```python
from build123d import *

# Parameters (mm, degrees)
SKETCH1_R                = 10
BOSS_EXTRUDE1_DEPTH      = 10
BOSS_EXTRUDE1_DEPTH_BACK = 10
SKETCH11_R               = 12.675
BOSS_EXTRUDE2_DEPTH      = 40
BOSS_EXTRUDE2_DEPTH_BACK = 40
SKETCH12_R               = 10.5
CUT_EXTRUDE6_DEPTH       = 81.0000001
SKETCH2_R                = 4.825
CUT_EXTRUDE7_DEPTH       = 30
LPATTERN1_COUNT          = 4
LPATTERN1_PITCH          = 4
LPATTERN2_COUNT          = 4
LPATTERN2_PITCH          = 4


with BuildPart() as part:
    # Sketch1 → Boss-Extrude1 (new body, two sides)
    with BuildSketch(Plane(origin=(0, 0, 0), x_dir=(0, 0, -1), z_dir=(1, 0, 0))) as boss_extrude1_sk:
        Circle(SKETCH1_R)
    extrude(amount=BOSS_EXTRUDE1_DEPTH)
    extrude(boss_extrude1_sk.sketch, amount=-BOSS_EXTRUDE1_DEPTH_BACK)

    # Sketch11 → Boss-Extrude2 (add, two sides)
    with BuildSketch(Plane.XY) as boss_extrude2_sk:
        with Locations((-17.400491433, 0)):
            Circle(SKETCH11_R)
    extrude(amount=BOSS_EXTRUDE2_DEPTH)
    extrude(boss_extrude2_sk.sketch, amount=-BOSS_EXTRUDE2_DEPTH_BACK)

    # Sketch12 → Cut-Extrude6 (cut, through all)
    with BuildSketch(Plane(origin=(0, 0, -40), x_dir=(-1, 0, 0), z_dir=(0, 0, -1))):
        with Locations((17.400491433, 0)):
            Circle(SKETCH12_R)
    extrude(amount=-CUT_EXTRUDE6_DEPTH, mode=Mode.SUBTRACT)

    # Sketch2 → Cut-Extrude7 (cut)
    with BuildSketch(Plane(origin=(10, 0, 0), x_dir=(0, 0, -1), z_dir=(1, 0, 0))):
        Circle(SKETCH2_R)
    extrude(amount=-CUT_EXTRUDE7_DEPTH, mode=Mode.SUBTRACT)

    # Sketch13 → Revolve1 (revolve)
    with BuildSketch(Plane.XY):
        Polygon((10, 4.825), (6, 4.825), (6, 4.325), align=None)
    revolve1 = revolve(axis=Axis((10, 0, 0), (-1, 0, 0)))

    # LPattern1: Revolve1 ×4
    with Locations(*[(-i * LPATTERN1_PITCH, 0, 0) for i in range(1, LPATTERN1_COUNT)]):
        add(revolve1)

    # Sketch17 → Revolve2 (revolve)
    with BuildSketch(Plane(origin=(-17.400491433, 0, 0), x_dir=(0, 0, -1), z_dir=(1, 0, 0))):
        Polygon((-40, 12.675), (-36, 12.675), (-36, 13.175), align=None)
    revolve2 = revolve(axis=Axis((-17.400491433, 0, 40), (0, 0, -1)))

    # LPattern2: Revolve2 ×4
    with Locations(*[(0, 0, -i * LPATTERN2_PITCH) for i in range(1, LPATTERN2_COUNT)]):
        add(revolve2)

    # Mirror1: Revolve2 across plane
    add(revolve2.mirror(Plane.XY))

    # Mirror1 copy 1 sketch → Mirror1 copy 1 (revolve)
    with BuildSketch(Plane(origin=(-17.400491433, 0, 4), x_dir=(0, 0, 1), z_dir=(1, 0, 0))):
        Polygon((-40, -12.675), (-36, -12.675), (-36, -13.175), align=None)
    revolve(axis=Axis((-17.400491433, 0, -36), (0, 0, -1)))

    # Mirror1 copy 2 sketch → Mirror1 copy 2 (revolve)
    with BuildSketch(Plane(origin=(-17.400491433, 0, 8), x_dir=(0, 0, 1), z_dir=(1, 0, 0))):
        Polygon((-40, -12.675), (-36, -12.675), (-36, -13.175), align=None)
    revolve(axis=Axis((-17.400491433, 0, -32), (0, 0, -1)))

    # Mirror1 copy 3 sketch → Mirror1 copy 3 (revolve)
    with BuildSketch(Plane(origin=(-17.400491433, 0, 12), x_dir=(0, 0, 1), z_dir=(1, 0, 0))):
        Polygon((-40, -12.675), (-36, -12.675), (-36, -13.175), align=None)
    revolve(axis=Axis((-17.400491433, 0, -28), (0, 0, -1)))


solid = part.part
```
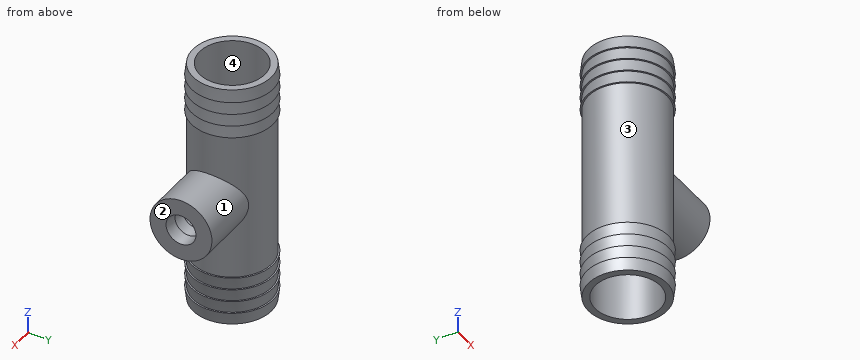
Model file for the job. Use its own axes, mm. Face numbers are marked on the shaded views. A direction names the side the tool comes from. Round coordinates to 2 decimals unless told otherwise and drop trailing zeros. Write each loop counter-clockwise with the first axis right and the second up, starting at its lowest first coordinate (ties: lowest second). Pieces come first, ordered by that corner, then holes. Notation, with made-up numbers: (-29, -36) -> (-24, -36) arc R21 ccw to (-24, -23) -> close; hole circle Ø4 at (58.25, 23.25). An arc over 180 degrees is marked (long way). Answer as CSV lines item,"result".
1. Slice it at B-B, the plane y = -2.25. State how many separate pieces and enclosed holes the cut face has, plus the area to 3 significant figures.
Resolved:
separate pieces,"3"
enclosed holes,"0"
area,"525 mm²"
2. Slice it at C-C, the plane x = 5. List the corners of the cut face in (y, z), plus the area to 3 significant figures.
Resolved:
outline,"circle Ø20 at (0, 0); hole circle Ø9.4 at (0, 0)"
area,"245 mm²"
3. Mould opens along Z. For the marked faces 3 and 4 say: +Z half, -Z half, draft (parallel to the pull), parting line (faces both ways), or undercut.
Resolved:
face 3,"undercut"
face 4,"draft"
4. Pin check, flat tips, straight feed: pin 1 Ø5 at (y, z) = (0.5, -1) entering from -X; pin 2 Ø12 at (x, z) = (-21.5, -9.5) entering from -Y (3 decimals); pin 3 Ø12 at (x, z) = (-17, -11) entering from +Y (3 decimals). Stop position of each tip, or through.
Resolved:
pin 1,"x = -30.08"
pin 2,"y = -12.675"
pin 3,"y = 12.675"
5. Tool access for the marked faces 1 and 2: list every direction of +Z, -Z, +X, -X, +Y, -Y with a clear straight run to the whole face (end or side of a thin tool).
Resolved:
face 1,"+X"
face 2,"+Z, -Z, +X, +Y, -Y"
6. Drill centre lines: line 1 (Z direction, x = -6.75, y = 0) (3 decimals); line 2 (Y direction, x = -7.15, z = 0) (3 decimals); line 3 (Z direction, x = -0.5, y = 2.5). Where is each one in solid material? Low to high.
Resolved:
line 1,"-40 to -4.825, 4.825 to 40"
line 2,"-10 to -4.825, 4.825 to 10"
line 3,"-9.68 to -3.76, 3.76 to 9.68"
